from build123d import *

# Parameters (mm, degrees)
ESQUISSE1_W                                 = 44
ESQUISSE1_H                                 = 44
BOSS_EXTRU_1_DEPTH                          = 1
FRAISAGE_POUR_VIS_T_TE_FRAIS_E_M21_AT_COUNT = 2
FRAISAGE_POUR_VIS_T_TE_FRAIS_E_M21_AT_PITCH = 39


with BuildPart() as part:
    # Esquisse1 → Boss.-Extru.1 (new body)
    with BuildSketch(Plane(origin=(0, 0, 0), x_dir=(0, 1, 0), z_dir=(0, 0, 1))):
        Rectangle(ESQUISSE1_W, ESQUISSE1_H)
    extrude(amount=BOSS_EXTRU_1_DEPTH)

    # Esquisse3 → Fraisage pour vis à tête fraisée M21 (revolve, cut)
    with BuildSketch(Plane(origin=(19.5, 19.5, 0), x_dir=(0, 1, 0), z_dir=(1, 0, 0))):
        Polygon((0, 0), (0, 2), (1.2, 2), (1.2, 1), (2.2, 0), align=None)
    fraisage_pour_vis_t_te_frais_e_m21 = revolve(axis=Axis((19.5, 19.5, -6.35), (0, 0, 1)), mode=Mode.SUBTRACT)

    # Fraisage pour vis à tête fraisée M21 at: Fraisage pour vis à tête fraisée M21 ×2
    with Locations(*[(-i * FRAISAGE_POUR_VIS_T_TE_FRAIS_E_M21_AT_PITCH, 0, 0) for i in range(1, FRAISAGE_POUR_VIS_T_TE_FRAIS_E_M21_AT_COUNT)]):
        add(fraisage_pour_vis_t_te_frais_e_m21, mode=Mode.SUBTRACT)

    # Symétrie2: Fraisage pour vis à tête fraisée M21 across plane
    add(fraisage_pour_vis_t_te_frais_e_m21.mirror(Plane.ZX), mode=Mode.SUBTRACT)

    # Symétrie2 copy 1 sketch → Symétrie2 copy 1 (revolve, cut)
    with BuildSketch(Plane(origin=(-19.5, -19.5, 0), x_dir=(0, -1, 0), z_dir=(1, 0, 0))):
        Polygon((0, 0), (0, -2), (1.2, -2), (1.2, -1), (2.2, 0), align=None)
    revolve(axis=Axis((-19.5, -19.5, -6.35), (0, 0, -1)), mode=Mode.SUBTRACT)


solid = part.part
Design review of the part built by this model. Coordinates are the model's own, in mm. Give positions to 0.01 mm unless a question says otherwise; leave off trailing zeros. Loops run counter-clockwise (first coordinate to the right, second up) from the corner with the lowest first, then second, coordinate; pieces in that order, holes last. Notation, with made-up numbers: (15, -25.75) -> (26, -25.75) arc R14 cw to (26, -18.75) -> close; hole circle Ø1 at (46, 18.5). An arc over 180 degrees is marked (long way). One line per question, with ' | ' between items. Start each with the question number.
(1) We need section B-B (x = -19.5). State the section outline as (y, z) points.
(2) For line 1 (Y direction, x = 18.5, z = 0.3); line 2 (Y direction, x = -18.5, z = 0.1); line 3 (X direction, y = 19, z = 0.95), list the stretches that pass through material, from the lowest coordinate up.
(3) We need section A-A (z = 0.15). State the section outline as (x, y) points.
The answers:
1) outline: (-22, 0) -> (-21.7, 0) -> (-20.7, 1) -> (-22, 1) -> close; (-18.3, 1) -> (-17.3, 0) -> (17.3, 0) -> (18.3, 1) -> close; (20.7, 1) -> (21.7, 0) -> (22, 0) -> (22, 1) -> close
2) line 1: y = -22 to -21.12, -17.88 to 17.88, 21.12 to 22 | line 2: y = -22 to -21.35, -17.65 to 17.65, 21.35 to 22 | line 3: x = -22 to -20.65, -18.35 to 18.35, 20.65 to 22
3) outline: (-22, -22) -> (22, -22) -> (22, 22) -> (-22, 22) -> close; hole circle Ø4.1 at (-19.5, -19.5); hole circle Ø4.1 at (-19.5, 19.5); hole circle Ø4.1 at (19.5, -19.5); hole circle Ø4.1 at (19.5, 19.5)
